```python
from build123d import *

# Parameters (mm, degrees)
EXTRUDE_1_DEPTH     = 7
SKETCH_3_W          = 8
SKETCH_3_H          = 7
EXTRUDE_3_DEPTH     = 13.5
SKETCH_2_R          = 2.5
SKETCH_2_R_2        = 1.999999991
CUT_EXTRUDE_2_DEPTH = 29.218856731
CHAMFER_1_SIZE      = 2


with BuildPart() as part:
    # Эскиз1 → Вытянуть1 (new body)
    with BuildSketch(Plane.XY):
        Polygon((-15, -1.146031522), (-15, -11.146031522), (15, -11.146031522), (15, -1.146031522), (4, -1.146031522), (4, 9.353968478), (-4, 9.353968478), (-4, -1.146031522), align=None)
    extrude(amount=EXTRUDE_1_DEPTH)

    # Эскиз3 → Вытянуть3 (add)
    with BuildSketch(Plane(origin=(0, 9.353968478, 0), x_dir=(1, 0, 0), z_dir=(0, 1, 0))):
        with Locations((0, -3.5)):
            Rectangle(SKETCH_3_W, SKETCH_3_H)
    extrude(amount=EXTRUDE_3_DEPTH)

    # Эскиз2 → Вытянуть2 (cut, through all)
    with BuildSketch(Plane.XY.offset(7)):
        with Locations((0, -1.14603177)):
            Circle(SKETCH_2_R)
        with Locations((4.2e-08, 11.794624395)):
            Circle(SKETCH_2_R_2)
    extrude(amount=-CUT_EXTRUDE_2_DEPTH, mode=Mode.SUBTRACT)

    # Фаска1
    chamfer_1_edges = [part.edges().sort_by_distance(p)[0] for p in [
        (4, 22.853968478, 3.5),
        (-4, 22.853968478, 3.5),
    ]]
    chamfer(chamfer_1_edges, length=CHAMFER_1_SIZE)


solid = part.part
```
Source: CAD feature listing. Evaluate the final solid. Frame: model axes, mm. A direction names the side the tool comes from. Coordinates: 2 decimals unless noted, no trailing zeros. Loops run counter-clockwise (first coordinate to the right, second up) from the corner with the lowest first, then second, coordinate; pieces in that order, holes last. Notation, with made-up numbers: (3.25, 25) -> (10.25, 25) arc R22 ccw to (10.25, 49) -> close; hole circle Ø5 at (11.5, 19.25). An arc over 180 degrees is marked (long way). One line per item, written item: value. Start each with the question number.
Q1. Section query C-C, the plane x = 6.5. Return the cut outline in (y, z).
Q2. Line query: line 1 along Y through (x, z) = (0, 3); line 2 along Y through (x, z) = (5.75, 5.5); line 3 along X through (y, z) = (10.5, 5.75). Output: solid intervals per line, ascending.
Q3. Set-up query: faces 4 (the face through (4, 10, 4)), 5 (the face through (-4, 10, 4)), 6 (the face through (0, 22.854, 3)). Return all of +Z, -Z, +X, -X, +Y, -Y with unobstructed straight access to the full face (end or side cutting, diameter ignored); none if empty.
Q4. Mould query, pull axis X, two halves, no side actions, for faces 1 (the face through (-9, -1.146, 3)), 2 (the face through (-0.542, -3.587, 3.549)), 3 (the face through (-2.986, 21.868, 3.549)). Classes: pulls with the +X half, pulls with the -X half, needs draft (parallel to the pull), parting line crosses it, or undercut.
Q5. Section query B-B, the plane z = 1.5. Return the cut outline in (x, y), and give its area (3 significant figures).
Q6. Contact query for flat-ended pins moving along their axis: P1, Ø5, axis at x = 12, y = 1.5, coming from the +Z side; P2, Ø3, axis at x = 4.5, z = 1, coming from the +Y side; P3, Ø3.5, axis at y = 13, z = 3.5, coming from the -X side; P4, Ø3.5, axis at x = 8, z = 2, coming from the +Y side. Output: stop coordinate, or through.
Q7. Section query D-D, the plane y = 20. Return the cut outline in (x, z).
Q8. Section query A-A, the plane x = 0. Return the cut outline in (y, z).
Results:
1. outline: (-11.15, 0) -> (-1.15, 0) -> (-1.15, 7) -> (-11.15, 7) -> close
2. line 1: -11.15 to -3.65, 1.35 to 9.79, 13.79 to 22.85
2. line 2: -11.15 to -1.15
2. line 3: -4 to -1.52, 1.52 to 4
3. face 4: +Z, -Z, +X, +Y
3. face 5: +Z, -Z, -X, +Y
3. face 6: +Z, -Z, +X, -X, +Y
4. face 1: needs draft
4. face 2: undercut
4. face 3: pulls with the -X half
5. outline: (-15, -11.15) -> (15, -11.15) -> (15, -1.15) -> (4, -1.15) -> (4, 20.85) -> (2, 22.85) -> (-2, 22.85) -> (-4, 20.85) -> (-4, -1.15) -> (-15, -1.15) -> close; hole circle Ø5 at (0, -1.15); hole circle Ø4 at (0, 11.79)
5. area: 456 mm^2
6. P1: through
6. P2: y = 21.85
6. P3: x = -4
6. P4: y = -1.15
7. outline: (-4, 0) -> (4, 0) -> (4, 7) -> (-4, 7) -> close
8. outline: (-11.15, 0) -> (-3.65, 0) -> (-3.65, 7) -> (-11.15, 7) -> close; (1.35, 0) -> (9.79, 0) -> (9.79, 7) -> (1.35, 7) -> close; (13.79, 0) -> (22.85, 0) -> (22.85, 7) -> (13.79, 7) -> close
